Geometry: final body of the model. Coordinates: model frame, mm. A direction names the side the tool comes from. Round coordinates to 2 decimals unless told otherwise and drop trailing zeros. Write each loop counter-clockwise with the first axis right and the second up, starting at its lowest first coordinate (ties: lowest second). Pieces come first, ordered by that corner, then holes. Notation, with made-up numbers: (-34.75, 53.5) -> (-12.75, 53.5) arc R16 cw to (-12.75, 64.5) -> close; hole circle Ø4 at (11, 1.25). An arc over 180 degrees is marked (long way). Use one line per item in the form item = value. Start each with the question number.
1. Line query: L1, parallel to Y at x = 1.5, z = -4.05 (3 decimals); L2, parallel to Y at x = 4.5, z = -0.8; L3, parallel to Z at x = 4.5, y = 17. Output: solid intervals per line, ascending.
2. Cut plane A-A, the plane x = 3.75. Return the cut outline in (y, z) (3 decimals).
3. Pin query (flat end, axial travel): pin 1 Ø0.7 at (x, y) = (4, -0.5) entering from +Z; pin 2 Ø1.1 at (x, y) = (4.5, 22) entering from -Z; pin 3 Ø1 at (x, z) = (5, -4.5) entering from +Y. Return the tip coordinate at first contact, or that it passes through.
4. Reachability of faces 5 (the face through (6, 10, 0)), 6 (the face through (0.5, 20.2, -5)), 7 (the face through (2.3, 21, -0.8)), 8 (the face through (7.98, 1.73, -4.12)), 9 (the face through (4, 21, -4)) from +Z, -Z, +X, -X, +Y, -Y: full face, straight path, thin tool, end or side. Return the list, or none.
5. Cut plane D-D, the plane x = 5.75. Return the cut outline in (y, z) (3 decimals), plus the area to 3 significant figures.
6. Cut plane B-B, the plane y = 20. Return the cut outline in (x, z), plus the area to 3 significant figures.
7. Draft query along Y for faces 1 (the face through (0.301, 0.74, -0.285)), 2 (the face through (2.3, 0, -0.8)), 3 (the face through (5, 11, -2)), 4 (the face through (3, 11, -5)). Return one class per face: pulls with the +Y half, pulls with the -Y half, needs draft (parallel to the pull), parting line crosses it, or undercut.
8. Cut plane C-C, the plane z = -3.1. Return the cut outline in (x, y) (3 decimals).
Autodesk Inventor part; units mm, degrees
ref_plane "YZ Plane" through (0, 0, 0) normal (1, 0, 0) x (0, 1, 0)
ref_plane "XZ Plane" through (0, 0, 0) normal (0, 1, 0) x (-1, 0, 0)
ref_plane "XY Plane" through (0, 0, 0) normal (0, 0, 1) x (1, 0, 0)
sketch "Эскиз1" plane through (0, 0, 0) normal (0, 1, 0) x (-1, 0, 0)
  line L0 (0, -5) -> (-1, -5)
  line L1 (-1, -5) -> (-3, -5)
  line L2 (-1, -5) -> (-6.5, -5)
  line L3 (-6.5, -5) -> (-6.5, -5)
  line L4 (0, -5) -> (0, -1)
  line L5 (-1, 0) -> (-6.5, 0)
  line L6 (-6.5, 0) -> (-6.5, -5)
  line L7 (-1, -5) -> (-1, -1.1)
  line L8 (-1.5, -0.6) -> (-6.5, -0.6)
  line L9 (-6.5, -0.6) -> (-6.5, -5)
  line L10 (-2, -5) -> (-2, -1.6)
  line L11 (-2, -1.6) -> (-5.5, -1.6)
  line L12 (-5.5, -1.6) -> (-5.5, -5.52)
  line L13 (-5.5, -1.6) -> (-6.5, -1.6)
  arc A0 (0, -1) -> (-1, 0) centre (-1, -1) ccw
  arc A1 (-1, -1.1) -> (-1.5, -0.6) centre (-1.5, -1.1) ccw
  point P0 (0, 0)
  point P1 (0, 0)
  point P2 (-1, -0.6)
  point P3 (-4.25, -5.52)
  dimension "d2" = 1
  dimension "d31" = 5
  dimension "d32" = 4.4
  dimension "d74" = 6.5
  dimension "d75" = 1
  dimension "d76" = 1
  dimension "d77" = 0.5
extrude "Выдавливание1" add sketch "Эскиз1" along normal blind 21
sketch "Эскиз2" plane through (0, 21, 0) normal (0, 1, 0) x (1, 0, 0)
  line L0 (6.5, 5.52) -> (1, 5.52)
  line L1 (1, 5.52) -> (1, 1.62)
  line L2 (1.5, 1.12) -> (6.5, 1.12)
  line L3 (6.5, 1.12) -> (6.5, 5.52)
  line L4 (6.5, 5) -> (0, 5)
  line L5 (2, 2.12) -> (2, 4.52)
  line L6 (2, 4.52) -> (5.5, 4.52)
  line L7 (5.5, 4.52) -> (5.5, 2.12)
  line L8 (5.5, 2.12) -> (2, 2.12)
  line L9 (6.5, 5.52) -> (2, 5.52)
  line L10 (2, 5.52) -> (2, 2.12)
  line L11 (2, 2.12) -> (6.5, 2.12)
  line L12 (6.5, 2.12) -> (6.5, 5.52)
  arc A0 (1, 1.62) -> (1.5, 1.12) centre (1.5, 1.62) ccw
  point P0 (0, 0)
  point P1 (1, 1.12)
  point P2 (2, 5)
  point P3 (1, 5)
  point P4 (2, 5.52)
  dimension "d78" = 5.5
  dimension "d79" = 4.4
  dimension "d80" = 0.52
  dimension "d81" = 1
  dimension "d82" = 0.5
extrude "Выдавливание2" add sketch "Эскиз2" along normal blind 1.425 and the other way blind 22.425 contours L10 L4 L1 L0 | L10 L5 L8 L11 L3 L2 A0 L1 L4
sketch "Эскиз6" plane through (0, 0, 0) normal (0, 0, 1) x (1, 0, 0)
  line L0 (0, 0) -> (0, 1.5)
  line L1 (0, 0) -> (0, 21)
  line L2 (0, 21) -> (6.5, 21)
  line L3 (0, 21) -> (0, 19.5)
  line L4 (0, 19.5) -> (5, 19.5)
  line L5 (5, 19.5) -> (5, 1.5)
  line L6 (5, 1.5) -> (0, 1.5)
  line L7 (0, 1.5) -> (0, 19.5)
  dimension "d33" = 1.5
  dimension "d34" = 1.5
  dimension "d35" = 5
extrude "Выдавливание5" cut sketch "Эскиз6" against normal blind 5
sketch "Эскиз7" plane through (6.5, 0, 0) normal (1, 0, 0) x (0, 0, -1)
  line L0 (0, 0) -> (0, 21)
  line L1 (2.12, 21) -> (5, 21)
  line L2 (0, 0) -> (5, 0)
  line L3 (5, 0) -> (5, 21)
  line L4 (5, 21) -> (0, 21)
  line L5 (0, 21) -> (0, 0)
  line L6 (5, 0) -> (5, 21)
  line L7 (0, 19.5) -> (0, 1.5)
  line L8 (4.52, 10.5) -> (4.52, 19.25)
  line L9 (4.52, 19.25) -> (4.52, 1.75)
  line L10 (5, 10.5) -> (0, 10.5)
  line L11 (4.52, 19.25) -> (4.52, 16.75)
  line L12 (4.52, 16.75) -> (4.52, 14.25)
  line L13 (4.52, 14.25) -> (4.52, 11.75)
  line L14 (4.52, 11.75) -> (4.52, 9.25)
  line L15 (4.52, 9.25) -> (4.52, 6.75)
  line L16 (4.52, 6.75) -> (4.52, 4.25)
  circle A0 centre (4.52, 4.25) radius 0.4
  circle A1 centre (4.52, 1.75) radius 0.4
  circle A2 centre (4.52, 9.25) radius 0.4
  circle A3 centre (4.52, 11.75) radius 0.4
  circle A4 centre (4.52, 14.25) radius 0.4
  circle A5 centre (4.52, 16.75) radius 0.4
  circle A6 centre (4.52, 19.25) radius 0.4
  line L17 (5.52, -1.425) -> (5.52, 22.425)
  dimension "d84" = 17.5
  dimension "d85" = 2.5
  dimension "d86" = 2.5
  dimension "d87" = 2.5
  dimension "d88" = 2.5
  dimension "d89" = 2.5
  dimension "d90" = 2.5
  dimension "d91" = 0.8
  dimension "d92" = 0.8
  dimension "d93" = 0.8
  dimension "d94" = 0.8
  dimension "d95" = 0.8
  dimension "d96" = 0.8
  dimension "d97" = 0.8
  dimension "d101" = 1
extrude "Выдавливание6" add sketch "Эскиз7" along normal blind 3 contours A1 | A0 L9 | L9 A0 | A2 L9 | L9 A2 | A6 | A5 L8 | L8 A5 | A4 L8 | L8 A4 | A3 L8 | L8 A3
ref_plane "РабПлоскость1" through (0, 10.5, 0) normal (0, 1, 0) x (1, 0, 0)
sketch "Эскиз10" plane through (0, 21, 0) normal (0, 1, 0) x (1, 0, 0)
  line L0 (6.5, 5) -> (2, 5)
  line L1 (2, 2.12) -> (2, 5.52)
  line L2 (6.5, 5) -> (2, 5)
  line L3 (2, 5) -> (2, 5.3)
  line L4 (2, 5.3) -> (6.5, 5.3)
  line L5 (6.5, 5.3) -> (6.5, 5)
  point P0 (0, 0)
  dimension "d98" = 0.3
extrude "Выдавливание7" add sketch "Эскиз10" against normal up to surface (21 mm away)
properties part number "battery_header 7P"
Outcome:
q1.L1 = -1.425 to 1.5, 19.5 to 22.425
q1.L2 = 0 to 1.5, 19.5 to 21
q1.L3 = -5.3 to -5
q2.outline = (-1.425, -2.12) -> (0, -2.12) -> (0, -5.3) -> (21, -5.3) -> (21, -2.12) -> (22.425, -2.12) -> (22.425, -1.12) -> (21, -1.12) -> (21, 0) -> (19.5, 0) -> (19.5, -5) -> (1.5, -5) -> (1.5, 0) -> (0, 0) -> (0, -1.12) -> (-1.425, -1.12) -> close
q3.pin_1 = -1.12
q3.pin_2 = -2.12
q3.pin_3 = 21
q4.face_5 = +Z, +X, -X, +Y, -Y
q4.face_6 = -Z, -X, +Y, -Y
q4.face_7 = +Z, -X, +Y
q4.face_8 = +X
q4.face_9 = -Z, +X, +Y
q5.outline = (-1.425, -2.12) -> (0, -2.12) -> (0, -5.3) -> (21, -5.3) -> (21, -2.12) -> (22.425, -2.12) -> (22.425, -1.12) -> (21, -1.12) -> (21, 0) -> (0, 0) -> (0, -1.12) -> (-1.425, -1.12) -> close
q5.area = 114 mm^2
q6.outline = (0, -5) -> (1, -5) -> (1, -5.52) -> (2, -5.52) -> (2, -5.3) -> (6.5, -5.3) -> (6.5, 0) -> (1, 0) arc R1 ccw to (0, -1) -> close
q6.area = 34.2 mm^2
q7.face_1 = needs draft
q7.face_2 = pulls with the -Y half
q7.face_3 = undercut
q7.face_4 = undercut
q8.outline = (0, 0) -> (1, 0) -> (1, -1.425) -> (2, -1.425) -> (2, 0) -> (6.5, 0) -> (6.5, 21) -> (2, 21) -> (2, 22.425) -> (1, 22.425) -> (1, 21) -> (0, 21) -> (0, 19.5) -> (5, 19.5) -> (5, 1.5) -> (0, 1.5) -> close
